The model under review builds one solid part; all positions refer to its coordinate system, in mm. Face numbers are marked on the shaded views. A direction names the side the tool comes from. Give positions to 0.01 mm unless a question says otherwise; leave off trailing zeros. Order: outer loops, then holes, each group sorted by start corner. A loop starts at its lowest first (then second) coordinate and runs counter-clockwise, first axis right, second up. Notation, with made-up numbers: (58.5, 13) - (70.5, 13) arc R16 ccw to (70.5, 32) - close; hole circle Ø10 at (72.5, -26). An arc over 180 degrees is marked (long way). Put each result on its own line as item: value.
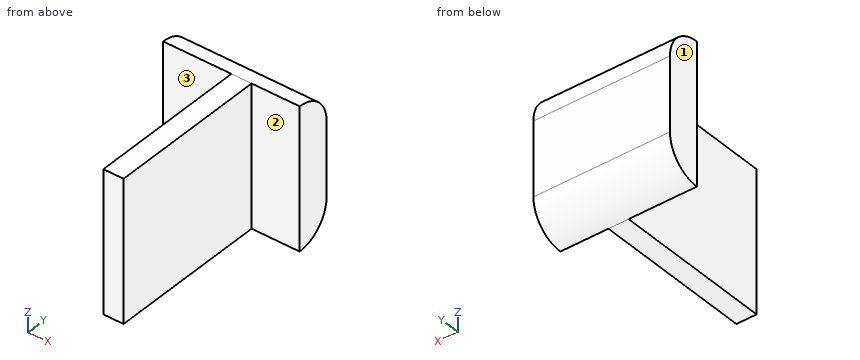
```python
from build123d import *

# Parameters (mm, degrees)
F1_E1_RIGHT_W = 20.9673028439
F1_E1_RIGHT_H = 23.7872338621
F2_DEPTH      = 3
F0_W          = 10.1448968053
F0_H          = 20.9673028439
F3_DEPTH      = 5
F4_R          = 5
F5_R          = 5


with BuildPart() as f2:
    # F1_E1_right (on explicit) → F2 (new body)
    with BuildSketch(Plane(origin=(-10.1448968053, 0, 16.1632616073), x_dir=(0, 0, 1), z_dir=(1, 0, 0))):
        with Locations((10.483651422, 11.893616931)):
            Rectangle(F1_E1_RIGHT_W, F1_E1_RIGHT_H)
    extrude(amount=F2_DEPTH)

    # F0 (on Front) → F3 (join)
    with BuildSketch(Plane.XZ):
        with Locations((-5.0724484026, 26.6469130293)):
            Rectangle(F0_W, F0_H)
        with Locations((-15.2173452079, 26.6469130293)):
            Rectangle(F0_W, F0_H)
    extrude(amount=-F3_DEPTH)

    # F4
    f4_edges = [f2.edges().sort_by_distance(p)[0] for p in [
        (-10.144897, 5, 37.130564),
    ]]
    fillet(f4_edges, radius=F4_R)

    # F5
    f5_edges = [f2.edges().sort_by_distance(p)[0] for p in [
        (-10.144897, 5, 16.163262),
    ]]
    fillet(f5_edges, radius=F5_R)


solid = f2.part
```
(1) Wall thickness on L1, parallel to X at y = -20.5, z = 29.75; L2, parallel to Y at x = -10.75, z = 23.5; L3, parallel to Y at x = -18.5, z = 17.75: over which ranges is each line inside the solid? List them lowest first.
The answers:
L1: -10.14 to -7.14
L2: 0 to 5
L3: 0 to 3.65
(2) Clearance check with flat-ended pins moving along their axes: pin 1 Ø8 at (y, z) = (-11, 18.5) entering from -X; pin 2 Ø6.5 at (y, z) = (-7.5, 27.5) entering from +X; pin 3 Ø2 at (x, z) = (-12, 28.5) entering from -Y; pin 4 Ø5 at (x, z) = (-7, 34.5) entering from +Y. State where each tip first meets the part, or that it passes through.
The answers:
pin 1: x = -10.14
pin 2: x = -7.14
pin 3: y = 0
pin 4: y = 5
(3) Take a section at A-A, the plane x = -9.5. Write out the cut boundary in (y, z).
The answers:
outline: (-23.79, 16.16) - (0, 16.16) arc R5 ccw to (5, 21.16) - (5, 32.13) arc R5 ccw to (0, 37.13) - (-23.79, 37.13) - close
(4) Take a section at D-D, the plane z = 19. Write out the cut boundary in (x, y).
The answers:
outline: (-20.29, 0) - (-10.14, 0) - (-10.14, -23.79) - (-7.14, -23.79) - (-7.14, 0) - (0, 0) - (0, 4.51) - (-20.29, 4.51) - close
(5) For the marked faces 1, 2 and 3, list the 3-axis set-ups (+Z, -Z, +X, -X, +Y, -Y) from which the entire face can be reached by the end or side of a thin tool; tool diameter is ignored.
The answers:
face 1: +Z, -Z, -X, +Y, -Y
face 2: +Z, -Z, +X, -Y
face 3: +Z, -Z, -X, -Y
(6) Take a section at C-C, the plane y = -8. Write out the cut boundary in (x, z), then the cut area to 3 significant figures.
The answers:
outline: (-10.14, 16.16) - (-7.14, 16.16) - (-7.14, 37.13) - (-10.14, 37.13) - close
area: 62.9 mm^2
(7) Take a section at B-B, the plane z = 30.75. Write out the cut boundary in (x, y).
The answers:
outline: (-20.29, 0) - (-10.14, 0) - (-10.14, -23.79) - (-7.14, -23.79) - (-7.14, 0) - (0, 0) - (0, 5) - (-20.29, 5) - close
